```python
from build123d import *

# Parameters (mm, degrees)
SKETCH_3_R      = 1.25
EXTRUDE_1_DEPTH = 1.7


with BuildPart() as part:
    # Эскиз3 → Бобышка-Вытянуть1 (new body)
    with BuildSketch(Plane.XY):
        with BuildLine():
            Line((-7.01136277, -24.439204164), (-6.594823284, -22.997133444))
            ThreePointArc((-6.594823284, -22.997133444), (-7.634692218, -19.522622744), (-11.227983542, -19.030881496))
            ThreePointArc((-11.227983542, -19.030881496), (-14.589641394, -19.446371526), (-17.557236321, -17.813351066))
            ThreePointArc((-17.557236321, -17.813351066), (0, 22.8), (17.557236321, -17.813351066))
            ThreePointArc((17.557236321, -17.813351066), (14.589641394, -19.446371526), (11.227983542, -19.030881496))
            ThreePointArc((11.227983542, -19.030881496), (7.634692218, -19.522622744), (6.594823284, -22.997133444))
            Line((6.594823284, -22.997133444), (7.01136277, -24.439204164))
            ThreePointArc((7.01136277, -24.439204164), (8.034444052, -25.671075647), (9.633424702, -25.757467432))
            ThreePointArc((9.633424702, -25.757467432), (0, 27.5), (-9.633424702, -25.757467432))
            ThreePointArc((-9.633424702, -25.757467432), (-8.034444052, -25.671075647), (-7.01136277, -24.439204164))
        make_face()
        with Locations((-9.813250738, -22.067496567)):
            Circle(SKETCH_3_R, mode=Mode.SUBTRACT)
        with Locations((9.813250738, -22.067496567)):
            Circle(SKETCH_3_R, mode=Mode.SUBTRACT)
    extrude(amount=EXTRUDE_1_DEPTH)


solid = part.part
```
Geometry: final body of the model. Coordinates: model frame, mm. A direction names the side the tool comes from. Round coordinates to 2 decimals unless told otherwise and drop trailing zeros. Write each loop counter-clockwise with the first axis right and the second up, starting at its lowest first coordinate (ties: lowest second). Pieces come first, ordered by that corner, then holes.
Item 1: Mould query, pull axis X, two halves, no side actions, for faces 3 (the face through (-4, 23, 1.7)), 4 (the face through (-14.542, -19.455, 0.838)), 5 (the face through (14.637, -19.437, 0.838)), 6 (the face through (1.07, 27.48, 0.84)). Classes: +X half, -X half, draft (parallel to the pull), parting line (faces both ways), or undercut.
Item 2: Section query D-D (x = 0). Return loops of the section in (y, z).
Item 3: Material intervals for L1, parallel to Y at x = 9.5, z = 0.15; L2, parallel to X at y = 5.5, z = 1.2; L3, parallel to Y at x = -15, z = 0.25, sorted ascending.
Item 4: Pin query (flat end, axial travel): P1, Ø3, axis at x = -19.5, y = 12.5, coming from the +Z side; P2, Ø1, axis at y = -20.5, z = 1.5, coming from the +X side. Return the tip coordinate at first contact, or that it passes through.
Item 5: Section query B-B (x = 14.5). Return loops of the section in (y, z), plus the area to 3 significant figures.
Item 6: Section query A-A (y = 6). Return loops of the section in (x, z), plus the area to 3 significant figures.
Item 7: Section query C-C (z = 0.7). Return loops of the section in (x, y).
Item 8: Set-up query: faces 1 (the face through (-6.806, -23.728, 0.838)), 2 (the face through (-7.59, -19.56, 0.84)). Return all of +Z, -Z, +X, -X, +Y, -Y with unobstructed straight access to the full face (end or side cutting, diameter ignored); none if empty.
Completed:
1. face 3: draft
1. face 4: undercut
1. face 5: undercut
1. face 6: parting line
2. outline: (22.8, 0) - (27.5, 0) - (27.5, 1.7) - (22.8, 1.7) - close
3. L1: y = -25.8 to -23.28, -20.86 to -18.73, 20.85 to 25.81
3. L2: x = -26.94 to -23.12, 23.12 to 26.94
3. L3: y = -23.05 to -19.35, 17.56 to 23.05
4. P1: stops at z = 1.7
4. P2: stops at x = 18.87
5. outline: (-23.37, 0) - (-19.46, 0) - (-19.46, 1.7) - (-23.37, 1.7) - close; (17.95, 0) - (23.37, 0) - (23.37, 1.7) - (17.95, 1.7) - close
5. area: 15.8 mm2
6. outline: (-26.84, 0) - (-22.97, 0) - (-22.97, 1.7) - (-26.84, 1.7) - close; (22.97, 0) - (26.84, 0) - (26.84, 1.7) - (22.97, 1.7) - close
6. area: 13.2 mm2
7. outline: (-17.56, -17.81) arc R24.1 cw (long way) to (17.56, -17.81) arc R5.5 cw to (11.23, -19.03) arc R3.35 ccw to (6.59, -23) - (7.01, -24.44) arc R2 ccw to (9.63, -25.76) arc R27.5 ccw (long way) to (-9.63, -25.76) arc R2 ccw to (-7.01, -24.44) - (-6.59, -23) arc R3.35 ccw to (-11.23, -19.03) arc R5.5 cw to start; hole circle Ø2.5 at (-9.81, -22.07); hole circle Ø2.5 at (9.81, -22.07)
8. face 1: +Z, -Z, -Y
8. face 2: +Z, -Z
